Check sheet for the drawn part. Datum: minimum x, y, z corner. Units: mm. Round coordinates to 2 decimals unless told otherwise and drop trailing zeros. Write each loop counter-clockwise with the first axis right and the second up, starting at its lowest first coordinate (ties: lowest second). Pieces come first, ordered by that corner, then holes. Notation, with made-up numbers: (17.5, 27.25) -> (31.5, 27.25) arc R10 ccw to (31.5, 40.25) -> close; hole circle Ø1 at (0, -30). An arc over 180 degrees is marked (long way). Use CSV: the item, a comma, the result in double quotes.
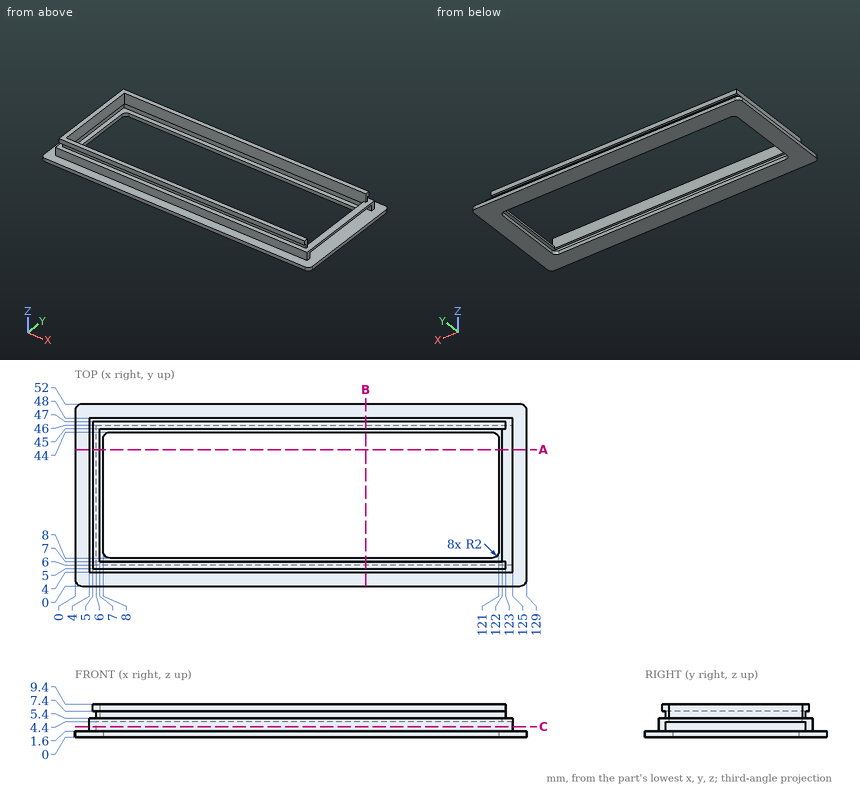
Q1. Material ranges on L1, parallel to Y at x = 57, z = 5; L2, parallel to Y at x = 48, z = 1.5; L3, parallel to X at y = 18.5, z = 5, recorded low to high.
Filled in:
L1,"4 to 7, 45 to 48"
L2,"0 to 8, 44 to 52"
L3,"4 to 7, 122 to 125"
Q2. Section check B-B (x = 83). Record the cut outline in (y, z), plus the area to 3 significant figures.
Filled in:
outline,"(0, 0) -> (8, 0) -> (8, 1.6) -> (6, 1.6) -> (6, 4.4) -> (7, 4.4) -> (7, 9.4) -> (5, 9.4) -> (5, 7.4) -> (6, 7.4) -> (6, 5.4) -> (4, 5.4) -> (4, 1.6) -> (0, 1.6) -> close; (44, 0) -> (52, 0) -> (52, 1.6) -> (48, 1.6) -> (48, 5.4) -> (46, 5.4) -> (46, 7.4) -> (47, 7.4) -> (47, 9.4) -> (45, 9.4) -> (45, 4.4) -> (46, 4.4) -> (46, 1.6) -> (44, 1.6) -> close"
area,"54.8 mm²"
Q3. Go/stop test with flat-tipped pins: P1, Ø0.6, axis at x = 70, z = 7, coming from the +Y side; P2, Ø2, axis at y = 22, z = 3.5, coming from the +X side; P3, Ø5.5, axis at x = 37.5, z = 7.5, coming from the +Y side; P4, Ø8, axis at x = 106.5, y = 13.5, coming from the -Z side. Record where each tip stops, or that it passes through.
Filled in:
P1,"y = 46"
P2,"x = 125"
P3,"y = 48"
P4,"through"
Q4. Section check A-A (y = 39). Record the cut outline in (x, z), plus the area to 3 significant figures.
Filled in:
outline,"(0, 0) -> (8, 0) -> (8, 1.6) -> (6, 1.6) -> (6, 4.4) -> (7, 4.4) -> (7, 9.4) -> (5, 9.4) -> (5, 7.4) -> (6, 7.4) -> (6, 5.4) -> (4, 5.4) -> (4, 1.6) -> (0, 1.6) -> close; (121, 0) -> (129, 0) -> (129, 1.6) -> (121, 1.6) -> close; (122, 4.4) -> (125, 4.4) -> (125, 5.4) -> (122, 5.4) -> close"
area,"43.2 mm²"
Q5. Section check C-C (z = 3). Record the cut outline in (x, y), plus the area to 3 significant figures.
Filled in:
outline,"(4, 4) -> (125, 4) -> (125, 6) -> (6, 6) -> (6, 46) -> (125, 46) -> (125, 48) -> (4, 48) -> close"
area,"564 mm²"
